```python
from build123d import *

# Parameters (mm, degrees)
SKETCH_1_R      = 7.5
EXTRUDE_1_DEPTH = 240
SKETCH_2_R      = 3.5
EXTRUDE_2_DEPTH = 13
SKETCH_3_R      = 3.5
EXTRUDE_3_DEPTH = 13
SKETCH_4_R      = 5
EXTRUDE_4_DEPTH = 2
SKETCH_5_R      = 5
EXTRUDE_5_DEPTH = 2


with BuildPart() as part:
    # 草图1 → 凸台-拉伸1 (new body)
    with BuildSketch(Plane.XY):
        Circle(SKETCH_1_R)
    extrude(amount=EXTRUDE_1_DEPTH)

    # 草图2 → 凸台-拉伸2 (add)
    with BuildSketch(Plane(origin=(0, 0, 0), x_dir=(-1, 0, 0), z_dir=(0, 0, -1))):
        Circle(SKETCH_2_R)
    extrude(amount=EXTRUDE_2_DEPTH)

    # 草图3 → 凸台-拉伸3 (add)
    with BuildSketch(Plane.XY.offset(240)):
        Circle(SKETCH_3_R)
    extrude(amount=EXTRUDE_3_DEPTH)

    # 草图4 → 凸台-拉伸4 (add)
    with BuildSketch(Plane(origin=(0, 0, 0), x_dir=(-1, 0, 0), z_dir=(0, 0, -1))):
        Circle(SKETCH_4_R)
    extrude(amount=EXTRUDE_4_DEPTH)

    # 草图5 → 凸台-拉伸5 (add)
    with BuildSketch(Plane.XY.offset(240)):
        Circle(SKETCH_5_R)
    extrude(amount=EXTRUDE_5_DEPTH)


solid = part.part
```
Verification items for the finished model (mm, model axes). A direction names the side the tool comes from. Give positions to 0.01 mm unless a question says otherwise; leave off trailing zeros. Loops run counter-clockwise (first coordinate to the right, second up) from the corner with the lowest first, then second, coordinate; pieces in that order, holes last. Notation, with made-up numbers: M 25.25,57.25 L 44.25,57.25 A8 ccw 44.25,61.25 Z; hole C 60.5,28 d7. An arc over 180 degrees is marked long. Return JSON: item names as keys, results as strings.
1) Material ranges on L1, parallel to Y at x = 0.75, z = 172.5; L2, parallel to Z at x = 3.5, y = -2.75; L3, parallel to Z at x = 6.25, y = -0.75, recorded low to high. Write a range as [from, to].
Findings:
{"L1": "y = [-7.46, 7.46]", "L2": "z = [-2, 242]", "L3": "z = [0, 240]"}
2) Section check C-C, the plane z = 233. Enter the section's corners in (x, y), and give its area (3 significant figures).
Findings:
{"outline": "C 0,0 d15", "area": "177 mm2"}
3) Tool access check on faces 1 (the flat face through (2, -5, 240)), 2 (the flat face through (0, 0, -13)), 3 (the cylindrical face through (1.08, -4.88, -0.99)). Record the directions out of +Z, -Z, +X, -X, +Y, -Y that give a thin tool (end or side, any length) a straight path to the whole face; none if there is none.
Findings:
{"face 1": "+Z", "face 2": "-Z, +X, -X, +Y, -Y", "face 3": "-Z"}
4) Section check A-A, the plane x = 0. Enter the section's corners in (y, z), and give its area (3 significant figures).
Findings:
{"outline": "M -7.5,0 L -5,0 L -5,-2 L -3.5,-2 L -3.5,-13 L 3.5,-13 L 3.5,-2 L 5,-2 L 5,0 L 7.5,0 L 7.5,240 L 5,240 L 5,242 L 3.5,242 L 3.5,253 L -3.5,253 L -3.5,242 L -5,242 L -5,240 L -7.5,240 Z", "area": "3,790 mm2"}
5) Gauge pin test, flat ends, axial feed: P1, Ø2, axis at x = -5, z = 101.5, coming from the +Y side; P2, Ø1, axis at y = -3.5, z = 90.5, coming from the +X side; P3, Ø3, axis at x = 3.5, z = 71, coming from the -Y side. Record the tip position at first contact, or that the pin passes through.
Findings:
{"P1": "stops at y = 6.34", "P2": "stops at x = 6.87", "P3": "stops at y = -7.23"}
